Can you work these out from the model? Positions are in its coordinate system, mm. Face numbers are marked on the shaded views. A direction names the side the tool comes from. Round coordinates to 2 decimals unless told otherwise and drop trailing zeros. Write each loop counter-clockwise with the first axis right and the second up, starting at its lowest first coordinate (ties: lowest second). Pieces come first, ordered by that corner, then holes.
Q1. If we section it at B-B (y = 25): Please give me the cut outline in (x, z), plus the area to 3 significant figures.
Q2. If we section it at A-A (y = 76.5): Please give me the cut outline in (x, z).
Q3. Please list where these lines run through material, in increasing order: line 1 along Z through (x, y) = (0, -5.95); line 2 along Y through (x, z) = (-17, 7) (3 decimals); line 3 along Y through (x, z) = (4.5, 21).
Q4. For the marked faces 5 and 6, which set-ups out of +Z, -Z, +X, -X, +Y, -Y let a thin tool reach every point of the face, with its end or its side?
Q5. We'd pull the mould along Z, two halves only. Please class the marked faces 1, 2, 3 and 4: +Z half, -Z half, draft (parallel to the pull), parting line (faces both ways), or undercut.
Q6. I'm going to push flat-ended pins straight in: pin 1 Ø3 at (x, z) = (13.5, -11) entering from +Y; pin 2 Ø1.9 at (x, z) = (15.18, -6.73) entering from -Y; pin 3 Ø1.6 at (x, y) = (-19, 1.5) entering from +Z. Where does each tip first touch, or does it pass through?
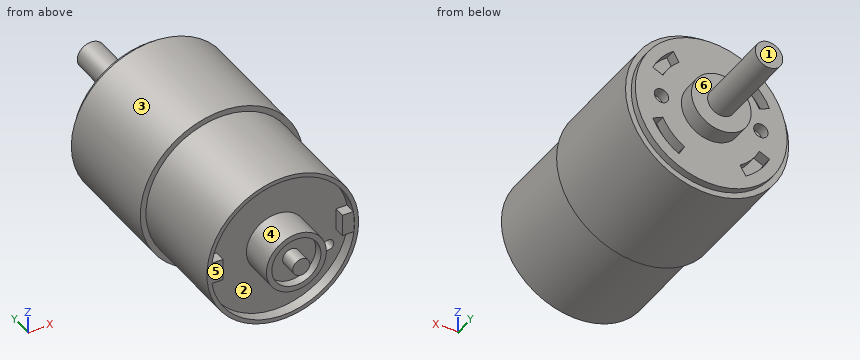
from build123d import *

# Parameters (mm, degrees)
SKETCH2_R            = 22.1488
BOSS_EXTRUDE4_DEPTH  = 66.0908
SKETCH4_R            = 8.6995
BOSS_EXTRUDE5_DEPTH  = 5.0038
SKETCH9_R            = 4.0005
BOSS_EXTRUDE6_DEPTH  = 23.5458
SKETCH10_R           = 8.7503
BOSS_EXTRUDE7_DEPTH  = 6.7056
SKETCH11_R           = 2.5019
BOSS_EXTRUDE8_DEPTH  = 2.413
SKETCH12_R           = 23.8125
BOSS_EXTRUDE9_DEPTH  = 34.0106
SKETCH13_R           = 2.0955
CUT_EXTRUDE1_DEPTH   = 3.175
CUT_EXTRUDE2_DEPTH   = 3.175
SKETCH15_R           = 20.958175
SKETCH15_R_2         = 8.7503
CUT_EXTRUDE3_DEPTH   = 3.175
SKETCH16_R           = 7.1628
SKETCH16_R_2         = 2.5019
CUT_EXTRUDE4_DEPTH   = 2.54
BOSS_EXTRUDE12_DEPTH = 3.175
BOSS_EXTRUDE13_DEPTH = 3.175
SKETCH20_R           = 1.5875
CUT_EXTRUDE5_DEPTH   = 3.175


with BuildPart() as part:
    # Sketch2 → Boss-Extrude4 (new body)
    with BuildSketch(Plane(origin=(0, 0, 0), x_dir=(1, 0, 0), z_dir=(0, 1, 0))):
        Circle(SKETCH2_R)
    extrude(amount=BOSS_EXTRUDE4_DEPTH)

    # Sketch4 → Boss-Extrude5 (add)
    with BuildSketch(Plane(origin=(0, 66.0908, 0), x_dir=(1, 0, 0), z_dir=(0, 1, 0))):
        Circle(SKETCH4_R)
    extrude(amount=BOSS_EXTRUDE5_DEPTH)

    # Sketch9 → Boss-Extrude6 (add)
    with BuildSketch(Plane(origin=(0, 71.0946, 0), x_dir=(1, 0, 0), z_dir=(0, 1, 0))):
        Circle(SKETCH9_R)
    extrude(amount=BOSS_EXTRUDE6_DEPTH)

    # Sketch10 → Boss-Extrude7 (add)
    with BuildSketch(Plane.XZ):
        Circle(SKETCH10_R)
    extrude(amount=BOSS_EXTRUDE7_DEPTH)

    # Sketch11 → Boss-Extrude8 (add)
    with BuildSketch(Plane.XZ.offset(6.7056)):
        Circle(SKETCH11_R)
    extrude(amount=BOSS_EXTRUDE8_DEPTH)

    # Sketch12 → Boss-Extrude9 (add)
    with BuildSketch(Plane(origin=(0, 64.0842, 0), x_dir=(-1, 0, 0), z_dir=(0, -1, 0))):
        Circle(SKETCH12_R)
    extrude(amount=BOSS_EXTRUDE9_DEPTH)

    # Sketch13 → Cut-Extrude1 (cut)
    with BuildSketch(Plane(origin=(0, 66.0908, 0), x_dir=(1, 0, 0), z_dir=(0, 1, 0))):
        with Locations((-14.5034, 0)):
            Circle(SKETCH13_R)
        with Locations((14.5034, 0)):
            Circle(SKETCH13_R)
    extrude(amount=-CUT_EXTRUDE1_DEPTH, mode=Mode.SUBTRACT)

    # Sketch14 → Cut-Extrude2 (cut)
    with BuildSketch(Plane(origin=(0, 66.0908, 0), x_dir=(1, 0, 0), z_dir=(0, 1, 0))):
        with BuildLine():
            Line((-14.070005184, -6.560951168), (-17.033311719, -7.942763698))
            ThreePointArc((-17.033311719, -7.942763698), (-13.856523006, -12.697163994), (-9.397090019, -16.276237356))
            Line((-9.397090019, -16.276237356), (-7.76226652, -13.444639995))
            ThreePointArc((-7.76226652, -13.444639995), (-11.445886375, -10.4882225), (-14.070005184, -6.560951168))
        make_face()
        with BuildLine():
            ThreePointArc((-10.080336815, 15.862156631), (-14.123267338, 12.399779151), (-17.033311719, 7.942763698))
            Line((-17.033311719, 7.942763698), (-14.070005184, 6.560951168))
            ThreePointArc((-14.070005184, 6.560951168), (-11.711998853, 10.190201616), (-8.44372295, 13.027458265))
            Line((-8.44372295, 13.027458265), (-10.080336815, 15.862156631))
        make_face()
        with BuildLine():
            ThreePointArc((17.033311719, 7.942763698), (13.856523006, 12.697163994), (9.397090019, 16.276237356))
            Line((9.397090019, 16.276237356), (7.76226652, 13.444639995))
            ThreePointArc((7.76226652, 13.444639995), (11.445886375, 10.4882225), (14.070005184, 6.560951168))
            Line((14.070005184, 6.560951168), (17.033311719, 7.942763698))
        make_face()
        with BuildLine():
            Line((9.385927189, -12.365900571), (11.031460095, -15.21604717))
            ThreePointArc((11.031460095, -15.21604717), (14.495965555, -11.961947414), (17.033311719, -7.942763698))
            Line((17.033311719, -7.942763698), (14.070005184, -6.560951168))
            ThreePointArc((14.070005184, -6.560951168), (12.081785889, -9.748926908), (9.385927189, -12.365900571))
        make_face()
    extrude(amount=-CUT_EXTRUDE2_DEPTH, mode=Mode.SUBTRACT)

    # Sketch15 → Cut-Extrude3 (cut)
    with BuildSketch(Plane.XZ):
        Circle(SKETCH15_R)
        Circle(SKETCH15_R_2, mode=Mode.SUBTRACT)
    extrude(amount=-CUT_EXTRUDE3_DEPTH, mode=Mode.SUBTRACT)

    # Sketch16 → Cut-Extrude4 (cut)
    with BuildSketch(Plane.XZ.offset(6.7056)):
        Circle(SKETCH16_R)
        Circle(SKETCH16_R_2, mode=Mode.SUBTRACT)
    extrude(amount=-CUT_EXTRUDE4_DEPTH, mode=Mode.SUBTRACT)

    # Sketch18 → Boss-Extrude12 (add)
    with BuildSketch(Plane.XZ):
        with BuildLine():
            ThreePointArc((20.865163654, 0), (20.780212376, 1.88091146), (20.52605029, 3.746506881))
            Line((20.52605029, 3.746506881), (17.399, 3.746506881))
            Line((17.399, 3.746506881), (17.399, -2.603493119))
            Line((17.399, -2.603493119), (20.702098393, -2.603493119))
            ThreePointArc((20.702098393, -2.603493119), (20.824357436, -1.304297387), (20.865163654, 0))
        make_face()
    extrude(amount=-BOSS_EXTRUDE12_DEPTH)

    # Sketch19 → Boss-Extrude13 (add)
    with BuildSketch(Plane(origin=(0, 0, 0), x_dir=(-1, 0, 0), z_dir=(0, -1, 0))):
        with BuildLine():
            Line((20.716285244, -3.175), (17.399, -3.175))
            Line((17.399, -3.175), (17.399, 3.175))
            Line((17.399, 3.175), (20.716285244, 3.175))
            ThreePointArc((20.716285244, 3.175), (20.958175, 0), (20.716285244, -3.175))
        make_face()
    extrude(amount=-BOSS_EXTRUDE13_DEPTH)

    # Sketch20 → Cut-Extrude5 (cut)
    with BuildSketch(Plane(origin=(0, 3.175, 0), x_dir=(-1, 0, 0), z_dir=(0, -1, 0))):
        with Locations((-15.1765, 6.730993119)):
            Circle(SKETCH20_R)
    extrude(amount=-CUT_EXTRUDE5_DEPTH, mode=Mode.SUBTRACT)


solid = part.part
A:
1. outline: circle Ø44.3 at (0, 0)
1. area: 1,540 mm2
2. outline: circle Ø8 at (0, 0)
3. line 1: z = -8.75 to -7.16, -2.5 to 2.5, 7.16 to 8.75
3. line 2: y = 3.175 to 66.091
3. line 3: y = 0 to 66.09
4. face 5: -Y
4. face 6: +Y
5. face 1: draft
5. face 2: undercut
5. face 3: parting line
5. face 4: undercut
6. pin 1: stops at y = 66.09
6. pin 2: stops at y = 6.35
6. pin 3: stops at z = 12.62
